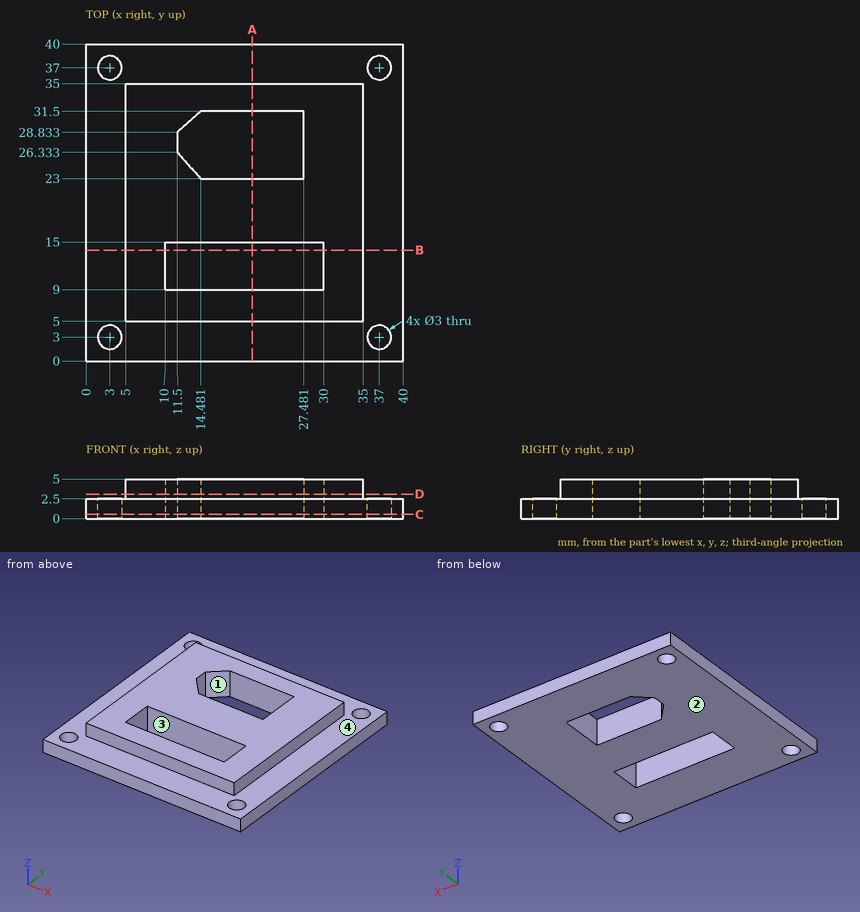
For this review, use the dimensioned drawing (mm, ordinates from the lowest corner) and the shaded views. A direction names the side the tool comes from. Coordinates: 2 decimals unless noted, no trailing zeros. Order: outer loops, then holes, each group sorted by start corner. A loop starts at its lowest first (then second) coordinate and runs counter-clockwise, first axis right, second up. Notation, with made-up numbers: M 70.25,11 L 106.25,11 A28 ccw 106.25,35 Z; hole C 36,-17 d9. An arc over 180 degrees is marked long. Answer as a JSON object with one key per item and string values. Group by question number.
1) Add section A-A, the plane x = 21. Write out the cut boundary in (y, z).
2) Wall thickness on L1, parallel to Y at x = 37, z = 1.1; L2, parallel to Y at x = 21, z = 0.6; L3, parallel to Y at x = 11, z = 3.8: over which ranges is each line inside the solid? List them lowest first.
3) Tool access review of the marked faces 1 and 2: name each direction out of +Z, -Z, +X, -X, +Y, -Y from which nothing blocks a thin tool from reaching the whole face with its end or side.
4) Mouldability with a two-part tool opening along Y and no side actions: class the marked faces 3 and 4 as pulls with the +Y half, pulls with the -Y half, needs draft (parallel to the pull), parting line crosses it, or undercut.
5) Add section D-D, the plane z = 3.1. Write out the cut boundary in (x, y), then the cut area to 3 significant figures.
6) Add section B-B, the plane y = 14. Write out the cut boundary in (x, z).
7) Add section C-C, the plane z = 0.55. Write out the cut boundary in (x, y).
8) For pin 1 (1.2 mm diameter, centred on y = 15, z = 3.5, fed in from -X); pin 2 (1 mm diameter, centred on x = 33.5, z = 3.5, fed in from +Y); pin 3 (2.5 mm diameter, centred on x = 37, y = 3, fed in from +Z); pin 4 (1.2 mm diameter, centred on x = 17.5, z = 3.5, fed in from -Y), all flat-tipped, find the tip position at first contact; note any pin that passes through.
Computed values:
{
 "1": {"outline": "M 0,0 L 9,0 L 9,5 L 5,5 L 5,2.5 L 0,2.5 Z; M 15,0 L 23,0 L 23,5 L 15,5 Z; M 31.5,0 L 40,0 L 40,2.5 L 35,2.5 L 35,5 L 31.5,5 Z"},
 "2": {"L1": "y = 0 to 1.5, 4.5 to 35.5, 38.5 to 40", "L2": "y = 0 to 9, 15 to 23, 31.5 to 40", "L3": "y = 5 to 9, 15 to 35"},
 "3": {"face 1": "+Z, -Z", "face 2": "-Z, +X, -X, +Y, -Y"},
 "4": {"face 3": "undercut", "face 4": "needs draft"},
 "5": {"outline": "M 5,5 L 35,5 L 35,35 L 5,35 Z; hole M 10,9 L 30,9 L 30,15 L 10,15 Z; hole M 11.5,26.33 L 14.48,23 L 27.48,23 L 27.48,31.5 L 14.48,31.5 L 11.5,28.83 Z", "area": "653 mm^2"},
 "6": {"outline": "M 0,0 L 10,0 L 10,5 L 5,5 L 5,2.5 L 0,2.5 Z; M 30,0 L 40,0 L 40,2.5 L 35,2.5 L 35,5 L 30,5 Z"},
 "7": {"outline": "M 0,0 L 40,0 L 40,40 L 0,40 Z; hole C 3,3 d3; hole C 3,37 d3; hole M 10,9 L 30,9 L 30,15 L 10,15 Z; hole M 11.5,26.33 L 14.48,23 L 27.48,23 L 27.48,31.5 L 14.48,31.5 L 11.5,28.83 Z; hole C 37,3 d3; hole C 37,37 d3"},
 "8": {"pin 1": "stops at x = 5", "pin 2": "stops at y = 35", "pin 3": "passes through", "pin 4": "stops at y = 5"}
}
